Autodesk Inventor part; units mm, degrees
ref_plane "YZ Plane" through (0, 0, 0) normal (1, 0, 0) x (0, 1, 0)
ref_plane "XZ Plane" through (0, 0, 0) normal (0, 1, 0) x (-1, 0, 0)
ref_plane "XY Plane" through (0, 0, 0) normal (0, 0, 1) x (1, 0, 0)
sketch "Sketch1" plane through (0, 0, 0) normal (0, 1, 0) x (-1, 0, 0)
  circle A0 centre (0, 0) radius 5
  arc A1 (5.25, 0) -> (-2.2187, -4.7581) centre (0, 0) ccw
  line L0 (-2.2187, -4.7581) -> (-8.4373, -1.8583)
  arc A2 (-8.4373, -1.8583) -> (-10.6939, -2.2562) centre (-9.2815, -3.6687) ccw
  line L1 (-10.6939, -2.2562) -> (-12.463, -4.0253)
  arc A3 (-12.463, -4.0253) -> (-11.0487, -5.4395) centre (-11.7558, -4.7324) ccw
  line L2 (-11.0487, -5.4395) -> (-9.281, -3.6717)
  line L3 (-9.281, -3.6717) -> (-3.064, -6.5707)
  arc A4 (-3.064, -6.5707) -> (6.0765, -3.9545) centre (0, 0) ccw
  line L4 (6.9147, -3.5) -> (9.4384, -3.5)
  line L5 (5.0312, -1.5) -> (10.9225, -1.5)
  line L6 (10.9384, -5) -> (10.9384, -12.2255)
  line L7 (10.9384, -12.2255) -> (-12.8, -12.2255)
  line L8 (10.9225, -1.5) -> (10.9225, 0)
  line L9 (12.0588, 0) -> (12.0588, -15.6375)
  line L10 (12.0588, -15.6375) -> (-14.9211, -15.6375)
  line L11 (0, 0) -> (7.7398, 0) construction
  line L12 (-12.8, -12.2255) -> (-14.9211, -15.6375)
  line L13 (10.9225, 0) -> (12.0588, 0)
  arc A5 (5.0312, -1.5) -> (5.25, 0) centre (0, 0) ccw
  arc A6 (-2.2187, -4.7581) -> (5.0312, -1.5) centre (0, 0) ccw
  arc A7 (10.9384, -5) -> (9.4384, -3.5) centre (9.4384, -5) ccw
  arc A8 (6.9147, -3.5) -> (6.0765, -3.9545) centre (6.9147, -4.5) ccw
  line L14 (-2.2187, 4.7581) -> (-8.4373, 1.8583)
  arc A9 (-10.6939, 2.2562) -> (-8.4373, 1.8583) centre (-9.2815, 3.6687) ccw
  line L15 (-10.6939, 2.2562) -> (-12.463, 4.0253)
  arc A10 (-11.0487, 5.4395) -> (-12.463, 4.0253) centre (-11.7558, 4.7324) ccw
  line L16 (-11.0487, 5.4395) -> (-9.281, 3.6717)
  line L17 (-9.281, 3.6717) -> (-3.064, 6.5707)
  arc A11 (6.0765, 3.9545) -> (-3.064, 6.5707) centre (0, 0) ccw
  line L18 (6.9147, 3.5) -> (9.4384, 3.5)
  line L19 (5.0312, 1.5) -> (10.9225, 1.5)
  line L20 (10.9384, 5) -> (10.9384, 12.2255)
  line L21 (10.9384, 12.2255) -> (-12.8, 12.2255)
  line L22 (10.9225, 1.5) -> (10.9225, 0)
  line L23 (12.0588, 0) -> (12.0588, 15.6375)
  line L24 (12.0588, 15.6375) -> (-14.9211, 15.6375)
  line L25 (-12.8, 12.2255) -> (-14.9211, 15.6375)
  arc A12 (5.0312, 1.5) -> (-2.2187, 4.7581) centre (0, 0) ccw
  arc A13 (9.4384, 3.5) -> (10.9384, 5) centre (9.4384, 5) ccw
  arc A14 (6.0765, 3.9545) -> (6.9147, 3.5) centre (6.9147, 4.5) ccw
  point P0 (6.3492, -3.5)
  point P1 (10.9384, -3.5)
  point P2 (6.3492, 3.5)
  point P3 (10.9384, 3.5)
  dimension "d0" = 10
  dimension "d1" = 10.5
  dimension "d2" = 2
  dimension "d3" = 2
  dimension "d4" = 2
  dimension "d5" = 25
  dimension "d6" = 1.5
  dimension "d7" = 110
  dimension "d8" = 2.5
  dimension "d11" = 1.5
  dimension "d12" = 1
extrude "Extrusion1" add sketch "Sketch1" along normal blind 10 contours A1 L14 A9 L15 A10 L16 L17 A11 A14 L18 A13 L20 L21 L25 L24 L23 L13 L22 L19 | L5 L8 L13 L9 L10 L12 L7 L6 A7 L4 A8 A4 L3 L2 A3 L1 A2 L0 A6
sketch "Sketch2" plane through (0, 0, 0) normal (0, -1, 0) x (1, 0, 0)
  line L0 (-10.9225, 1.5) -> (-10.9225, -1.5)
  line L1 (-5.0312, 1.5) -> (-10.9225, 1.5)
  arc A0 (2.2187, 4.7581) -> (-5.0312, 1.5) centre (0, 0) ccw
  line L2 (8.4373, 1.8583) -> (2.2187, 4.7581)
  arc A1 (8.4373, 1.8583) -> (10.6939, 2.2562) centre (9.2815, 3.6687) ccw
  line L3 (12.463, 4.0253) -> (10.6939, 2.2562)
  arc A2 (12.463, 4.0253) -> (11.0487, 5.4395) centre (11.7558, 4.7324) ccw
  line L4 (9.281, 3.6717) -> (11.0487, 5.4395)
  line L5 (3.064, 6.5707) -> (9.281, 3.6717)
  arc A3 (3.064, 6.5707) -> (-6.0765, 3.9545) centre (0, 0) ccw
  arc A4 (-6.9147, 3.5) -> (-6.0765, 3.9545) centre (-6.9147, 4.5) ccw
  line L6 (-9.4384, 3.5) -> (-6.9147, 3.5)
  arc A5 (-10.9384, 5) -> (-9.4384, 3.5) centre (-9.4384, 5) ccw
  line L7 (-10.9384, 12.2255) -> (-10.9384, 5)
  line L8 (12.8, 12.2255) -> (-10.9384, 12.2255)
  line L9 (14.9211, 15.6375) -> (12.8, 12.2255)
  line L10 (-12.0588, 15.6375) -> (14.9211, 15.6375)
  line L11 (-12.0588, -15.6375) -> (-12.0588, 15.6375)
  line L12 (14.9211, -15.6375) -> (-12.0588, -15.6375)
  line L13 (12.8, -12.2255) -> (14.9211, -15.6375)
  line L14 (-10.9384, -12.2255) -> (12.8, -12.2255)
  line L15 (-10.9384, -5) -> (-10.9384, -12.2255)
  arc A6 (-9.4384, -3.5) -> (-10.9384, -5) centre (-9.4384, -5) ccw
  line L16 (-6.9147, -3.5) -> (-9.4384, -3.5)
  arc A7 (-6.0765, -3.9545) -> (-6.9147, -3.5) centre (-6.9147, -4.5) ccw
  arc A8 (-6.0765, -3.9545) -> (3.064, -6.5707) centre (0, 0) ccw
  line L17 (9.281, -3.6717) -> (3.064, -6.5707)
  line L18 (11.0487, -5.4395) -> (9.281, -3.6717)
  arc A9 (11.0487, -5.4395) -> (12.463, -4.0253) centre (11.7558, -4.7324) ccw
  line L19 (10.6939, -2.2562) -> (12.463, -4.0253)
  arc A10 (10.6939, -2.2562) -> (8.4373, -1.8583) centre (9.2815, -3.6687) ccw
  line L20 (2.2187, -4.7581) -> (8.4373, -1.8583)
  arc A11 (-5.0312, -1.5) -> (2.2187, -4.7581) centre (0, 0) ccw
  line L21 (-10.9225, -1.5) -> (-5.0312, -1.5)
  arc A12 (-9.4384, -3.5) -> (-10.9384, -5) centre (-9.4384, -5) ccw
  line L22 (-10.9384, 5) -> (-10.9384, -5)
extrude "Extrusion2" add sketch "Sketch2" along normal blind 3 contours L22 L15 L14 L13 L12 L11 L10 L9 L8 L7
sketch "Sketch3" plane through (0, -3, 0) normal (0, -1, 0) x (1, 0, 0)
  line L0 (14.9211, -15.6375) -> (12.8, -12.2255)
  line L1 (-12.0588, 15.6375) -> (14.9211, 15.6375)
  line L2 (14.9211, 15.6375) -> (14.9211, -15.6375)
  line L3 (14.9211, -15.6375) -> (-12.0588, -15.6375)
  line L4 (-12.0588, -15.6375) -> (-12.0588, 15.6375)
  point P0 (0, 0)
extrude "Extrusion3" add sketch "Sketch3" along normal blind 2
properties part number "shaft holder clip"
CAD build for the part. Positions are in the model's coordinates, mm. A direction names the side the tool comes from. Round coordinates to 2 decimals unless told otherwise and drop trailing zeros. Loops run counter-clockwise (first coordinate to the right, second up) from the corner with the lowest first, then second, coordinate; pieces in that order, holes last.
(1) Cut at D-D (x = -1). Give the cut face in (y, z).
(2) Cut at B-B (x = 4). Give the cut face in (y, z).
(3) Which spindle directions (+Z, -Z, +X, -X, +Y, -Y) get a long thin tool onto all of the face, cutting with end or side? Do faces 5 (the flat face through (2, 3, -15.638)), 6 (the flat face through (-8, 5, 1.5)), 7 (the cylindrical face through (9.61, 4.93, 1.7)), 8 (the flat face through (5, 10, 4)), 9 (the flat face through (2, -3, 0)). Say none if no direction does.
(4) Drop flat-ended pins along their axis: pin 1 (0.9 mm diameter, centred on y = 3.5, z = -0.5, fed in from +X); pin 2 (4 mm diameter, centred on y = 5.5, z = 7, fed in from +X); pin 3 (2 mm diameter, centred on y = 8, z = 4.5, fed in from +X). Give the stop position or say it passes through.
(5) Wall check: line 1 along Z through (x, y) = (-9.5, 0.5); line 2 along Z through (x, y) = (-0.25, 4); line 3 along X through (y, z) = (5, 4). Give the ranges that are in metal, low to high.
(6) Two-plate mould, pull along X, no slides. Class faces 1 (the cylindrical face through (-6.432, 4.93, -3.624)), 2 (the flat face through (-8, 5, -1.5)), 3 (the flat face through (-10.922, 5, 0)), 4 (the cylindrical face through (-10.49, 4.93, -3.93)): +X half, -X half, draft (parallel to the pull), parting line (faces both ways), or undercut.
Findings below:
1. outline: (-5, -15.64) - (10, -15.64) - (10, -12.23) - (-3, -12.23) - (-3, 12.23) - (10, 12.23) - (10, 15.64) - (-5, 15.64) - close; (0, -7.18) - (10, -7.18) - (10, -5.15) - (0, -5.15) - close; (0, 5.15) - (10, 5.15) - (10, 7.18) - (0, 7.18) - close
2. outline: (-5, -15.64) - (10, -15.64) - (10, -12.23) - (-3, -12.23) - (-3, 12.23) - (10, 12.23) - (10, 15.64) - (-5, 15.64) - close; (0, -6.13) - (10, -6.13) - (10, -3.93) - (0, -3.93) - close; (0, 3.93) - (10, 3.93) - (10, 6.13) - (0, 6.13) - close
3. face 5: -Z, +X, -X, +Y, -Y
3. face 6: +X, +Y
3. face 7: +Y
3. face 8: +Z, -Z, +X, -X, +Y
3. face 9: +X
4. pin 1: stops at x = -10.92
4. pin 2: stops at x = 12.72
4. pin 3: stops at x = 12.76
5. line 1: z = -15.64 to -12.23, -3.5 to -1.5, 1.5 to 3.5, 12.23 to 15.64
5. line 2: z = -15.64 to -12.23, -7.25 to -5.24, 5.24 to 7.25, 12.23 to 15.64
5. line 3: x = -12.06 to -10.56, -6.05 to -3.4, 3.84 to 8.58, 9.61 to 12.44
6. face 1: undercut
6. face 2: draft
6. face 3: +X half
6. face 4: undercut
